Source: CAD feature listing. Evaluate the final solid. Frame: model axes, mm. A direction names the side the tool comes from. Give positions to 0.01 mm unless a question says otherwise; leave off trailing zeros. Write each loop counter-clockwise with the first axis right and the second up, starting at its lowest first coordinate (ties: lowest second). Pieces come first, ordered by that corner, then holes. Notation, with made-up numbers: (43, 83.5) - (57, 83.5) arc R26 cw to (57, 116.5) - close; hole circle Ø6 at (72.25, -14.5). An arc over 180 degrees is marked (long way). One line per question, with ' | ' between items. Start each with the question number.
(1) Draft query along Y for faces 1 (the cylindrical face through (-1.5, 0.07, 4.93)), 2 (the cylindrical face through (-3.87, 2.226, 5.07)), 3 (the flat face through (12, 2, 40)), 4 (the cylindrical face through (0.007, -4.464, 25.07)). Return one class per face: +Y half, -Y half, draft (parallel to the pull), parting line (faces both ways), or undercut.
(2) Section C-C, the plane y = 0. Return loops of the section in (x, z).
(3) Ray query, line 1 (Z direction, x = 12.5, y = 3.9); line 2 (X direction, y = 0.75, z = 7.5); line 3 (X direction, y = -0.25, z = 6.5). Return the intervals inside material, ascending. Write a range as [from, to].
(4) Access query for faces 5 (the flat face through (4, -1, 5)), 6 (the flat face through (-4, 0, 25)), 7 (the flat face through (5, 2, 15)), 8 (the flat face through (-2.021, -3.452, 4.93)), 9 (the flat face through (5, 2, 35)). Directions: +Z, -Z, +X, -X, +Y, -Y. A direction counts if a zero-diameter tool reaches every point of the face in a straight line with its end or side. Return the directions, or none.
(5) Section B-B, the plane x = 12.5. Return loops of the section in (y, z), plus the area to 3 significant figures.
(6) Pin query (flat end, axial travel): pin 1 (2.5 mm diameter, centred on y = 2.5, z = 13, fed in from -X); pin 2 (1.1 mm diameter, centred on y = -1, z = 24.5, fed in from +X); pin 3 (2 mm diameter, centred on x = 11, y = -3, fed in from +Z); pin 4 (7 mm diameter, centred on x = 12.5, z = 32.5, fed in from -Y). Return the tip coordinate at first contact, or that it passes through.
(7) Section A-A, the plane z = 7.5. Return loops of the section in (x, y).
(8) Section D-D, the plane x = -1. Return loops of the section in (y, z), plus the area to 3 significant figures.
```python
from build123d import *

# Parameters (mm, degrees)
SKETCH1_R      = 1.5
EXTRUDE1_DEPTH = 40
SKETCH2_R      = 2.75
EXTRUDE2_DEPTH = 10
CHAMFER1_SIZE  = 2
SKETCH3_W      = 12.733635698
SKETCH3_H      = 10
SKETCH3_W_2    = 13.399455213
EXTRUDE3_DEPTH = 10
FILLET1_R      = 1


with BuildPart() as part:
    # Sketch1 → Extrude1 (new body)
    with BuildSketch(Plane.XY):
        Polygon((4, -0.381197846), (17.5, -0.381197846), (20, 2.118802154), (20, 4.618802154), (0, 4.618802154), (-4, 2.309401077), (-4, -2.309401077), (0, -4.618802154), (4, -2.309401077), align=None)
        Circle(SKETCH1_R, mode=Mode.SUBTRACT)
    extrude(amount=EXTRUDE1_DEPTH)

    # Sketch2 → Extrude2 (cut)
    with BuildSketch(Plane.XZ.offset(0.381197846)):
        with Locations((12.5, 32.5)):
            Circle(SKETCH2_R)
        with Locations((12.5, 7.5)):
            Circle(SKETCH2_R)
    extrude(amount=-EXTRUDE2_DEPTH, mode=Mode.SUBTRACT)

    # Chamfer1
    chamfer1_edges = [part.edges().sort_by_distance(p)[0] for p in [
        (9.75, -0.381197846, 32.5),
        (9.75, -0.381197846, 7.5),
    ]]
    chamfer(chamfer1_edges, length=CHAMFER1_SIZE)

    # Sketch3 → Extrude3 (cut)
    with BuildSketch(Plane(origin=(0, 4.618802154, 0), x_dir=(1, 0, 0), z_dir=(0, 1, 0))):
        with Locations((-1.366817849, -35)):
            Rectangle(SKETCH3_W, SKETCH3_H)
        with Locations((-1.699727607, -15)):
            Rectangle(SKETCH3_W_2, SKETCH3_H)
    extrude(amount=-EXTRUDE3_DEPTH, mode=Mode.SUBTRACT)

    # Fillet1
    fillet1_edges = [part.edges().sort_by_distance(p)[0] for p in [
        (4, -2.309401077, 25),
        (4, -2.309401077, 5),
        (0, -4.618802154, 25),
        (0, -4.618802154, 5),
        (-4, -2.309401077, 25),
        (-4, -2.309401077, 5),
        (-4, 2.309401077, 25),
        (-4, 2.309401077, 5),
        (0, 4.618802154, 25),
        (0, 4.618802154, 5),
    ]]
    fillet(fillet1_edges, radius=FILLET1_R)


solid = part.part
```
Check sheet entries:
1) face 1: undercut | face 2: +Y half | face 3: draft | face 4: -Y half
2) outline: (-4, 0) - (-1.5, 0) - (-1.5, 10) - (-4, 10) - close; (-4, 20) - (-1.5, 20) - (-1.5, 30) - (-4, 30) - close; (1.5, 0) - (17.88, 0) - (17.88, 40) - (5, 40) - (5, 30) - (1.5, 30) - (1.5, 20) - (5, 20) - (5, 10) - (1.5, 10) - close; hole circle Ø8.74 at (12.5, 7.5); hole circle Ø8.74 at (12.5, 32.5)
3) line 1: [0, 4.75], [10.25, 29.75], [35.25, 40] | line 2: [-4, -1.3], [1.3, 8.88], [16.12, 18.63] | line 3: [-4, -1.48], [1.48, 7.99], [17.01, 17.63]
4) face 5: +Z, -Z, +X, -Y | face 6: +Z, -Z, -X, +Y, -Y | face 7: -X, +Y, -Y | face 8: +Z, -Z, -X, -Y | face 9: +Z, -X, +Y, -Y
5) outline: (-0.38, 0) - (4.62, 0) - (4.62, 4.75) - (1.62, 4.75) - (-0.38, 2.75) - close; (-0.38, 12.25) - (1.62, 10.25) - (4.62, 10.25) - (4.62, 29.75) - (1.62, 29.75) - (-0.38, 27.75) - close; (-0.38, 37.25) - (1.62, 35.25) - (4.62, 35.25) - (4.62, 40) - (-0.38, 40) - close | area: 137 mm²
6) pin 1: x = 5 | pin 2: x = 4 | pin 3: through | pin 4: y = 0.87
7) outline: (-4, -1.73) arc R1 ccw to (-3.5, -2.6) - (-0.5, -4.33) arc R1 ccw to (0.5, -4.33) - (3.5, -2.6) arc R1 ccw to (4, -1.73) - (4, -0.38) - (7.75, -0.38) - (9.75, 1.62) - (9.75, 4.62) - (0.27, 4.62) arc R1 ccw to (-0.23, 4.48) - (-3.5, 2.6) arc R1 ccw to (-4, 1.73) - close; (15.25, 1.62) - (17.25, -0.38) - (17.5, -0.38) - (20, 2.12) - (20, 4.62) - (15.25, 4.62) - close; hole circle Ø3 at (0, 0)
8) outline: (-4.04, 0) - (-1.12, 0) - (-1.12, 10) - (-4.04, 10) - close; (-4.04, 20) - (-1.12, 20) - (-1.12, 30) - (-4.04, 30) - close; (1.12, 0) - (4.04, 0) - (4.04, 10) - (1.12, 10) - close; (1.12, 20) - (4.04, 20) - (4.04, 30) - (1.12, 30) - close | area: 117 mm²
